from build123d import *

# Parameters (mm, degrees)
SKETCH1_R           = 2
SKETCH1_R_2         = 2.5
BOSS_EXTRUDE1_DEPTH = 16
SKETCH2_R           = 4
BOSS_EXTRUDE2_DEPTH = 10


with BuildPart() as part:
    # Sketch1 → Boss-Extrude1 (new body)
    with BuildSketch(Plane.XY):
        with BuildLine():
            Line((0, 15), (45, 15))
            Line((45, 15), (45, -15))
            Line((45, -15), (0, -15))
            ThreePointArc((0, -15), (-15, 0), (0, 15))
        make_face()
        with Locations((40, 10)):
            Circle(SKETCH1_R, mode=Mode.SUBTRACT)
        with Locations((40, -10)):
            Circle(SKETCH1_R, mode=Mode.SUBTRACT)
        Circle(SKETCH1_R_2, mode=Mode.SUBTRACT)
    extrude(amount=BOSS_EXTRUDE1_DEPTH)

    # Sketch2 → Boss-Extrude2 (add)
    with BuildSketch(Plane(origin=(45, 0, 0), x_dir=(0, 0, -1), z_dir=(1, 0, 0))):
        with Locations(Location((-8.334071627, 0, 0), (0, 0, 270))):
            Circle(SKETCH2_R)
    extrude(amount=BOSS_EXTRUDE2_DEPTH)


solid = part.part
Read the model definition and answer for the solid it produces. Units are mm, in the model's axes. A direction names the side the tool comes from. Give positions to 0.01 mm unless a question says otherwise; leave off trailing zeros. Write each loop counter-clockwise with the first axis right and the second up, starting at its lowest first coordinate (ties: lowest second). Pieces come first, ordered by that corner, then holes. Notation, with made-up numbers: (-19, -14.5) -> (-4, -14.5) arc R26 ccw to (-4, 23.5) -> close; hole circle Ø5 at (83, 36). An arc over 180 degrees is marked (long way). Answer as a JSON object with one key per item and string values. Group by question number.
1) Find section A-A (x = 40). Write down the section's boundary in (y, z).
2) Find section C-C (z = 1.75). Write down the section's boundary in (x, y).
3) Consider L1, parallel to Y at x = 0, z = 7.75; L2, parallel to Y at x = 40, z = 5.5; L3, parallel to X at y = 11, z = 12.75. Determine where each line is inside the solid, lowest interval first. Write a range as from..to.
4) Find section B-B (y = 0). Write down the section's boundary in (x, z).
5) Find section D-D (x = 1.5). Write down the section's boundary in (y, z).
6) A tool of negligible diameter and unlimited length cuts with its end or side. For faces 4 (the cylindrical face through (49.93, 3.174, 10.768)), 5 (the cylindrical face through (38.526, 11.352, 7.888)), from which of +Z, -Z, +X, -X, +Y, -Y can it reach the whole face along a straight path? Write none if from no direction.
7) The mould has two halves that part along X. Classify faces 1 (the flat face through (15, 0, 16)), 2 (the cylindrical face through (-0.54, -2.44, 7.89)), 3 (the flat face through (55, 0, 8)): +X half, -X half, draft (parallel to the pull), parting line (faces both ways), or undercut.
8) Each of these flat-tipped pins is pushed along its axis until it touches: P1, Ø3, axis at y = -5.5, z = 4.5, coming from the -X side; P2, Ø2, axis at y = -2, z = 13.5, coming from the -X side; P3, Ø8, axis at y = -11, z = 13, coming from the +X side. Where does it stop, or does it pass through?
Values follow:
{
 "1": {"outline": "(-15, 0) -> (-12, 0) -> (-12, 16) -> (-15, 16) -> close; (-8, 0) -> (8, 0) -> (8, 16) -> (-8, 16) -> close; (12, 0) -> (15, 0) -> (15, 16) -> (12, 16) -> close"},
 "2": {"outline": "(0, -15) -> (45, -15) -> (45, 15) -> (0, 15) arc R15 ccw to start; hole circle Ø5 at (0, 0); hole circle Ø4 at (40, -10); hole circle Ø4 at (40, 10)"},
 "3": {"L1": "y = -15..-2.5, 2.5..15", "L2": "y = -15..-12, -8..8, 12..15", "L3": "x = -10.2..38.27, 41.73..45"},
 "4": {"outline": "(-15, 0) -> (-2.5, 0) -> (-2.5, 16) -> (-15, 16) -> close; (2.5, 0) -> (45, 0) -> (45, 4.33) -> (55, 4.33) -> (55, 12.33) -> (45, 12.33) -> (45, 16) -> (2.5, 16) -> close"},
 "5": {"outline": "(-15, 0) -> (-2, 0) -> (-2, 16) -> (-15, 16) -> close; (2, 0) -> (15, 0) -> (15, 16) -> (2, 16) -> close"},
 "6": {"face 4": "+X", "face 5": "+Z, -Z"},
 "7": {"face 1": "draft", "face 2": "undercut", "face 3": "+X half"},
 "8": {"P1": "stops at x = -14.46", "P2": "stops at x = -14.97", "P3": "stops at x = 45"}
}
